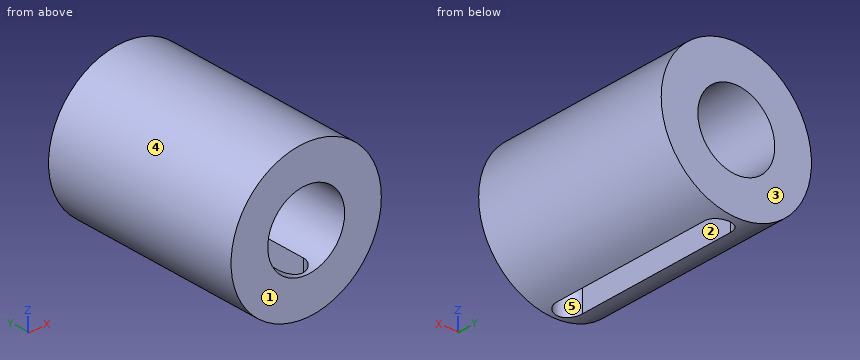
from build123d import *

# Parameters (mm, degrees)
SKETCH1_W          = 14.417582417
SKETCH1_H          = 80
CUT_EXTRUDE1_DEPTH = 30.538461538


with BuildPart() as part:
    # Sketch1 → Revolve1 (revolve)
    with BuildSketch(Plane.XY):
        with Locations((22.32967033, 6.065934066)):
            Rectangle(SKETCH1_W, SKETCH1_H)
    revolve(axis=Axis((0, 46.065934066, 0), (0, -1, 0)))

    # Sketch2 → Cut-Extrude1 (cut, through all)
    with BuildSketch(Plane.XY):
        with BuildLine():
            Line((5.140001029, 37.869690433), (5.140001029, -27.129905913))
            ThreePointArc((5.140001029, -27.129905913), (0, -32.269906942), (-5.140001029, -27.129905913))
            Line((-5.140001029, -27.129905913), (-5.140001029, 37.869690433))
            ThreePointArc((-5.140001029, 37.869690433), (0, 43.009691462), (5.140001029, 37.869690433))
        make_face()
    extrude(amount=-CUT_EXTRUDE1_DEPTH, mode=Mode.SUBTRACT)


solid = part.part
Could you check a few things on this model? Use its own coordinates, in mm. Face numbers are marked on the shaded views. A direction names the side the tool comes from. Give positions to 0.01 mm unless a question says otherwise; leave off trailing zeros. Order: outer loops, then holes, each group sorted by start corner. A loop starts at its lowest first (then second) coordinate and runs counter-clockwise, first axis right, second up. Notation, with made-up numbers: (44.5, 85) -> (55.5, 85) arc R22 cw to (55.5, 122) -> close; hole circle Ø1 at (-26, 44). An arc over 180 degrees is marked (long way). Answer in a Markdown table with one row per item. Add a question column.
Item 1: Please list where these lines run through material, in increasing order: probe 1 along X at (y, z) = (-5.5, -0.5); probe 2 along Z at (x, y) = (0, 6); probe 3 along X at (y, z) = (-10, -11.5).
Item 2: For the marked faces 4 and 5, which set-ups out of +Z, -Z, +X, -X, +Y, -Y let a thin tool reach every point of the face, with its end or its side?
Item 3: Imagine slicing it at B-B (z = 0). List the corners of the cut face in (x, y) for me.
Item 4: Imagine slicing it at C-C (z = -24.5). List the corners of the cut face in (x, y) for me, and give its area (3 significant figures).
Item 5: I'm going to push flat-ended pins straight in: P1, Ø12, axis at y = 0, z = -18, coming from the -X side; P2, Ø8, axis at y = 36, z = 20.5, coming from the -X side; P3, Ø2, axis at x = -7.5, y = 2, coming from the +Z side; P4, Ø6, axis at x = 21, z = -23, coming from the -Y side. Where does each tip first touch, or does it pass through?
Item 6: Imagine slicing it at D-D (y = -10). List the corners of the cut face in (x, z) for me.
Item 7: Imagine slicing it at A-A (x = 0). List the corners of the cut face in (y, z) for me.
Item 8: We'd pull the mould along Y, two halves only. Please class the marked faces 1, 2 and 3: pulls with the +Y half, pulls with the -Y half, needs draft (parallel to the pull), parting line crosses it, or undercut.
Result:
| question | item | result |
|---|---|---|
| 1 | probe 1 | -29.53 to -15.11, 15.11 to 29.53 |
| 1 | probe 2 | 15.12 to 29.54 |
| 1 | probe 3 | -27.21 to -9.82, 9.82 to 27.21 |
| 2 | face 4 | +Y, -Y |
| 2 | face 5 | -Z |
| 3 | outline | (-29.54, -33.93) -> (-15.12, -33.93) -> (-15.12, 46.07) -> (-29.54, 46.07) -> close; (15.12, -33.93) -> (29.54, -33.93) -> (29.54, 46.07) -> (15.12, 46.07) -> close |
| 4 | outline | (-16.5, -33.93) -> (16.5, -33.93) -> (16.5, 46.07) -> (-16.5, 46.07) -> close; hole (-5.14, -27.13) arc R5.14 ccw to (5.14, -27.13) -> (5.14, 37.87) arc R5.14 ccw to (-5.14, 37.87) -> close |
| 4 | area | 1,890 mm2 |
| 5 | P1 | x = -26.99 |
| 5 | P2 | x = -24.5 |
| 5 | P3 | z = 28.81 |
| 5 | P4 | y = -33.93 |
| 6 | outline | (-5.14, -29.09) -> (-5.14, -14.22) arc R15.12 cw (long way) to (5.14, -14.22) -> (5.14, -29.09) arc R29.54 ccw (long way) to start |
| 7 | outline | (-33.93, -29.54) -> (-32.27, -29.54) -> (-32.27, -15.12) -> (-33.93, -15.12) -> close; (-33.93, 15.12) -> (46.07, 15.12) -> (46.07, 29.54) -> (-33.93, 29.54) -> close; (43.01, -29.54) -> (46.07, -29.54) -> (46.07, -15.12) -> (43.01, -15.12) -> close |
| 8 | face 1 | pulls with the -Y half |
| 8 | face 2 | undercut |
| 8 | face 3 | pulls with the +Y half |
